For this review, take the finished solid that the model builds, in its own axes (mm). A direction names the side the tool comes from. Round coordinates to 2 decimals unless told otherwise and drop trailing zeros. Loops run counter-clockwise (first coordinate to the right, second up) from the corner with the lowest first, then second, coordinate; pieces in that order, holes last. Notation, with made-up numbers: M 61.5,69.25 L 86.5,69.25 A14 cw 86.5,93.25 Z; hole C -30.75,45.25 d5. An arc over 180 degrees is marked long. One line per question, with ' | ' between items. Start each with the question number.
1) We need section A-A (z = 38). Give the boundary of the cut face in (x, y), and give its area (3 significant figures).
2) For probe 1 along X at (y, z) = (4, 0); probe 2 along Y at (x, z) = (-3.5, -57); probe 3 along Z at (x, y) = (-0.25, 13), list the stretches that pass through material, from the lowest coordinate up. Write a range as from..to.
3) For faces 4 (the face through (2.253, 6.902, 7.154)), 5 (the face through (-3.2, 14, 3.2)), list the 3-axis set-ups (+Z, -Z, +X, -X, +Y, -Y) from which the entire face can be reached by the end or side of a thin tool; tool diameter is ignored.
4) For pin 1 Ø1.5 at (x, z) = (3, -58) entering from +Y; pin 2 Ø6 at (x, y) = (-4, 6.5) entering from +Z; pin 3 Ø5 at (x, z) = (2.5, -26) entering from +Y, all flat-tipped, find the tip position at first contact; note any pin that passes through.
5) Mouldability with a two-part tool opening along X and no side actions: class faces 1 (the face through (4.214, 7.098, -0.553)), 2 (the face through (-3.2, 0, 3.2)), 3 (the face through (4.49, 5.79, -111.49)) as pulls with the +X half, pulls with the -X half, needs draft (parallel to the pull), parting line crosses it, or undercut.
```python
from build123d import *

# Parameters (mm, degrees)
SKETCH1_R           = 7.5
BOSS_EXTRUDE2_DEPTH = 14
CUT_EXTRUDE1_REACH  = 19.564
SKETCH2_R           = 4.25
BOSS_EXTRUDE3_START = -7.279118874
BOSS_EXTRUDE3_DEPTH = 1.03527618
FILLET1_R           = 10
CIRPATTERN1_COUNT   = 2
FILLET3_R           = 10


with BuildPart() as part:
    # Sketch1 → Boss-Extrude2 (new body)
    with BuildSketch(Plane(origin=(0, 0, 0), x_dir=(1, 0, 0), z_dir=(0, 1, 0))):
        with Locations(Location((0, 0, 0), (0, 0, 270))):
            Circle(SKETCH1_R)
    extrude(amount=BOSS_EXTRUDE2_DEPTH)

    # Sketch2 → Cut-Extrude1 (cut, up to next)
    with BuildSketch(Plane(origin=(0, 14, 0), x_dir=(1, 0, 0), z_dir=(0, 1, 0)), mode=Mode.PRIVATE) as cut_extrude1_sk1:
        with Locations(Location((0, 0, 0), (0, 0, 270))):
            Circle(SKETCH2_R)
    cut_extrude1_tool1 = extrude(cut_extrude1_sk1.sketch, amount=-CUT_EXTRUDE1_REACH, mode=Mode.PRIVATE) & part.part
    add(cut_extrude1_tool1.solids().sort_by_distance((0, 14, 0))[0], mode=Mode.SUBTRACT)

    # Boss-Extrude3: read off the stored shape, not the designer's step
    # Boss-Extrude3 outline → Boss-Extrude3 (add)
    with BuildSketch(Plane(origin=(0, 0, 0), x_dir=(0.9659258262890672, 0.2588190451025251, 0), z_dir=(0.25881904510252507, -0.9659258262890672, 0)).offset(BOSS_EXTRUDE3_START)):
        with BuildLine():
            add(Edge.make_bspline(
                [(-5.688266684, 1.344969698), (-4.547659305, 7.389056985), (1.811733316, 7.498803292)],
                knots=[0.18030465, 0.18030465, 0.18030465, 1.551469461, 1.551469461, 1.551469461], degree=2, weights=[1, 0.771122328, 0.993637519]))
            add(Edge.make_bspline(
                [(1.811733316, 7.498803292), (8.171125936, 7.389056985), (9.311733316, 1.344969698)],
                knots=[1.590123193, 1.590123193, 1.590123193, 2.961288004, 2.961288004, 2.961288004], degree=2, weights=[0.993637519, 0.771122328, 1]))
            Line((9.311733316, 1.344969698), (9.311733316, 114.5))
            Line((9.311733316, 114.5), (-5.688266684, 114.5))
            Line((-5.688266684, 114.5), (-5.688266684, 1.344969698))
        make_face()
    boss_extrude3 = extrude(amount=BOSS_EXTRUDE3_DEPTH)

    # Fillet1
    fillet1_edges = [part.edges().sort_by_distance(p)[0] for p in [
        (-7.244443697, 5.058857162, 114.5),
    ]]
    fillet(fillet1_edges, radius=FILLET1_R)

    # CirPattern1: Boss-Extrude3 ×2 about axis
    cirpattern1_axis = Axis((0, 0, 0), (0, 1, 0))
    for i in range(1, CIRPATTERN1_COUNT):
        add(boss_extrude3.rotate(cirpattern1_axis, i * 360 / CIRPATTERN1_COUNT))

    # Fillet3
    fillet3_edges = [part.edges().sort_by_distance(p)[0] for p in [
        (7.244443697, 5.058857162, -114.5),
    ]]
    fillet(fillet3_edges, radius=FILLET3_R)


solid = part.part
```
Answers below:
1) outline: M -7.38,5.56 L -7.11,4.56 L 7.38,8.44 L 7.11,9.44 Z | area: 15.5 mm^2
2) probe 1: -7.5..-4.25, 4.25..7.5 | probe 2: 7.4..8.47 | probe 3: -7.5..-4.24, 4.24..7.5
3) face 4: none | face 5: +Z, -Z, +X, -X, +Y
4) pin 1: y = 6.93 | pin 2: z = 113.87 | pin 3: y = 7.54
5) face 1: undercut | face 2: needs draft | face 3: pulls with the +X half
